Can you work these out from the drawing? Everything is in mm from the part's minimum corner. Give positions to 0.01 mm unless a question says otherwise; leave off trailing zeros. Order: outer loops, then holes, each group sorted by start corner. A loop starts at its lowest first (then second) coordinate and runs counter-clockwise, first axis right, second up. Notation, with made-up numbers: M 9.25,-8.5 L 33.25,-8.5 A11 cw 33.25,3.5 Z; hole C -36.75,53 d8. An arc over 180 degrees is marked long. Answer as a JSON object with one key per item and string values.
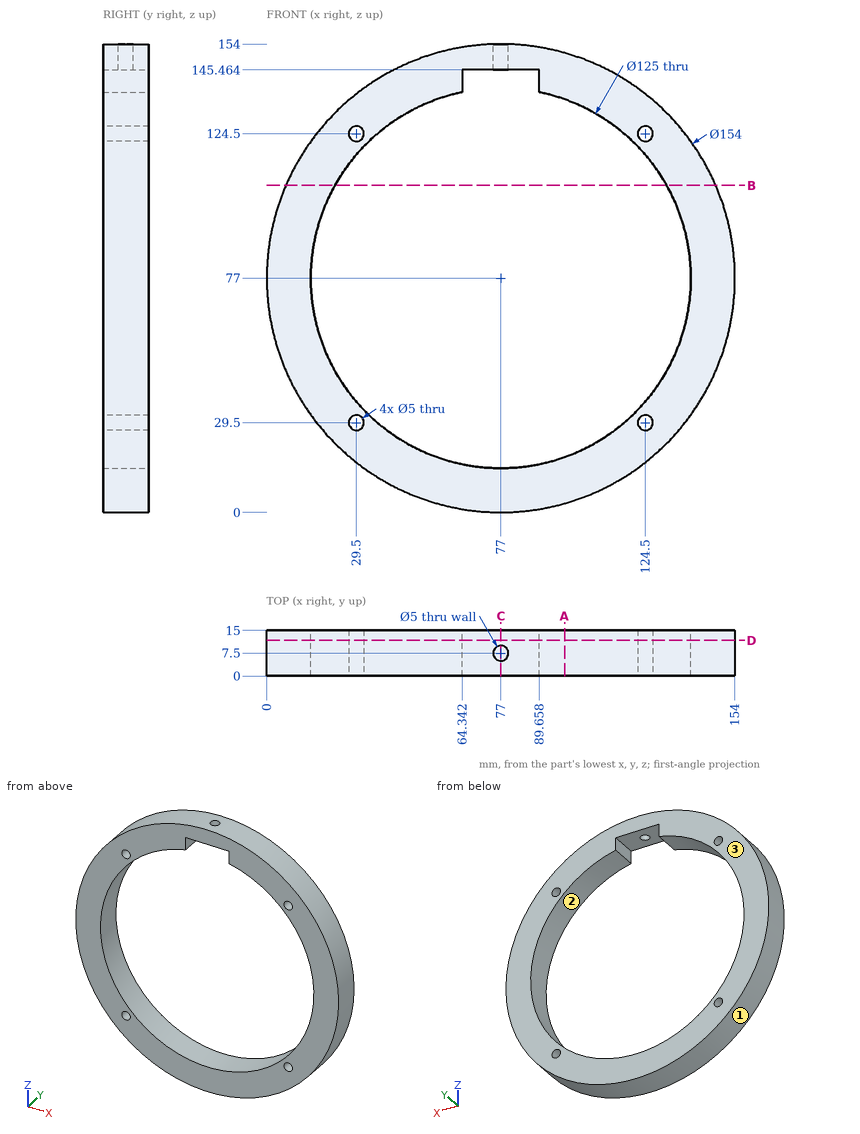
1) I want a section at D-D on y = 11.75. Write out the boundary of the cut face in (x, z) (1 decimal), and give its area (3 significant figures).
Results found:
{"outline": "C 77,77 d154; hole C 29.5,29.5 d5; hole C 29.5,124.5 d5; hole M 64.3,138.2 A62.5 ccw long 89.7,138.2 L 89.7,145.5 L 64.3,145.5 Z; hole C 124.5,29.5 d5; hole C 124.5,124.5 d5", "area": "6,110 mm²"}
2) I want a section at B-B on z = 107.5. Write out the boundary of the cut face in (x, y).
Results found:
{"outline": "M 6.3,0 L 22.45,0 L 22.45,15 L 6.3,15 Z; M 131.55,0 L 147.7,0 L 147.7,15 L 131.55,15 Z"}
3) I want a section at A-A on x = 98. Write out the boundary of the cut face in (y, z).
Results found:
{"outline": "M 0,2.92 L 15,2.92 L 15,18.13 L 0,18.13 Z; M 0,135.87 L 15,135.87 L 15,151.08 L 0,151.08 Z"}
4) Thinking about a two-plate mould opening in Z: for the marked faces 1, 2 and 3, which applies, pulls with the +Z half, pulls with the -Z half, needs draft (parallel to the pull), parting line crosses it, or undercut?
Results found:
{"face 1": "parting line crosses it", "face 2": "undercut", "face 3": "needs draft"}
5) I'm going to push flat-ended pins straight in: pin 1 Ø5 at (x, y) = (133.5, 4.5) entering from -Z; pin 2 Ø6 at (x, y) = (80.5, 4) entering from +Z; pin 3 Ø8 at (y, z) = (6, 141.5) entering from +X; pin 4 Ø4.5 at (x, z) = (29.5, 124.5) entering from -Y. Where does each tip first touch, or does it pass through?
Results found:
{"pin 1": "stops at z = 22.11", "pin 2": "stops at z = 154", "pin 3": "stops at x = 124.63", "pin 4": "passes through"}
6) I need wall thicknesses on L1, parallel to Y at x = 77, z = 149; L2, parallel to Z at x = 124.5, y = 8.25 (1 decimal); L3, parallel to Z at x = 116, y = 6.5. Which ranges of each line are inside material? Lowest first, please.
Results found:
{"L1": "y = 0 to 5, 10 to 15", "L2": "z = 16.4 to 27, 32 to 36.4, 117.6 to 122, 127 to 137.6", "L3": "z = 10.61 to 28.16, 125.84 to 143.39"}
7) I want a section at C-C on x = 77. Write out the boundary of the cut face in (y, z), and give its area (3 significant figures).
Results found:
{"outline": "M 0,0 L 15,0 L 15,14.5 L 0,14.5 Z; M 0,145.46 L 5,145.46 L 5,154 L 0,154 Z; M 10,145.46 L 15,145.46 L 15,154 L 10,154 Z", "area": "303 mm²"}
